```python
from build123d import *

# Parameters (mm, degrees)
REDONDEO1_R = 0.2


with BuildPart() as part:
    # Croquis2 → Revolución1 (revolve)
    with BuildSketch(Plane(origin=(0, 0, 0), x_dir=(1, 0, 0), z_dir=(0, 1, 0))):
        Polygon((0, 0), (0, 3), (0.5, 3), (0.5, 4), (0, 4), (0, 15.5), (-2.25, 15.5), (-2.25, 17.5), (3, 17.5), (3, 0), align=None)
    revolve(axis=Axis((3, 0, -17.5), (0, 0, 1)))

    # Redondeo1
    redondeo1_edges = [part.edges().sort_by_distance(p)[0] for p in [
        (8.25, 0, -17.5),
        (8.25, 0, -15.5),
    ]]
    fillet(redondeo1_edges, radius=REDONDEO1_R)


solid = part.part
```
Work out the finished part from the listing and answer in its coordinate system (mm). A direction names the side the tool comes from. Round coordinates to 2 decimals unless told otherwise and drop trailing zeros. Loops run counter-clockwise (first coordinate to the right, second up) from the corner with the lowest first, then second, coordinate; pieces in that order, holes last. Notation, with made-up numbers: (39, -5.75) -> (53, -5.75) arc R10 cw to (53, 3.25) -> close; hole circle Ø1 at (49, 26). An arc over 180 degrees is marked (long way). Write each question's results on one line, items separated by ' | '. Start each with the question number.
1. Given pin 1 Ø3 at (y, z) = (-3.5, -9) entering from +X; pin 2 Ø2 at (x, z) = (0.5, -14) entering from +Y; pin 3 Ø5 at (x, y) = (2.5, -1) entering from +Z; pin 4 Ø3 at (y, z) = (-1.5, -14.5) entering from +X, each flat-ended and moving along its own axis, determine where each tip first touches the part or whether it passes through.
2. Section C-C (z = -3.5) is taken. Determine the outline of the cut face in (x, y).
3. A tool of negligible diameter and unlimited length cuts with its end or side. For faces 1 (the face through (1, -2, -4)), 2 (the face through (2.9, 3.3, -15.5)), 3 (the face through (8.245, -0.231, -16.511)), from which of +Z, -Z, +X, -X, +Y, -Y can it reach the whole face along a straight path? Write none if from no direction.
4. Find the intervals of material crossed by probe 1 along Z at (x, y) = (5.25, 3); probe 2 along Y at (x, z) = (5, -13.5); probe 3 along X at (y, z) = (-2, -16.5), in increasing order. Write a range as from..to.
5. Section B-B (x = 3) is taken. Determine the outline of the cut face in (y, z).
6. For a pull along Z with two mould halves and no side action, classify faces 4 (the face through (3, 0, -17.5)), 5 (the face through (5, -2, -3)), 6 (the face through (5.4, 1.8, -9.8)) as +Z half, -Z half, draft (parallel to the pull), parting line (faces both ways), or undercut.
7. Section A-A (y = 0) is taken. Determine the outline of the cut face in (x, z), plus the area to 3 significant figures.
Evaluation:
1) pin 1: stops at x = 5.24 | pin 2: stops at y = 2.6 | pin 3: stops at z = 0 | pin 4: stops at x = 8.22
2) outline: circle Ø5 at (3, 0)
3) face 1: none | face 2: +Z | face 3: +Z, -Z
4) probe 1: z = -17.5..-15.5 | probe 2: y = -2.24..2.24 | probe 3: x = -1.85..7.85
5) outline: (-5.25, -17.3) arc R0.2 ccw to (-5.05, -17.5) -> (5.05, -17.5) arc R0.2 ccw to (5.25, -17.3) -> (5.25, -15.7) arc R0.2 ccw to (5.05, -15.5) -> (3, -15.5) -> (3, -4) -> (2.5, -4) -> (2.5, -3) -> (3, -3) -> (3, 0) -> (-3, 0) -> (-3, -3) -> (-2.5, -3) -> (-2.5, -4) -> (-3, -4) -> (-3, -15.5) -> (-5.05, -15.5) arc R0.2 ccw to (-5.25, -15.7) -> close
6) face 4: -Z half | face 5: undercut | face 6: draft
7) outline: (-2.25, -17.3) arc R0.2 ccw to (-2.05, -17.5) -> (8.05, -17.5) arc R0.2 ccw to (8.25, -17.3) -> (8.25, -15.7) arc R0.2 ccw to (8.05, -15.5) -> (6, -15.5) -> (6, -4) -> (5.5, -4) -> (5.5, -3) -> (6, -3) -> (6, 0) -> (0, 0) -> (0, -3) -> (0.5, -3) -> (0.5, -4) -> (0, -4) -> (0, -15.5) -> (-2.05, -15.5) arc R0.2 ccw to (-2.25, -15.7) -> close | area: 113 mm2
